Check sheet for the drawn part. Datum: minimum x, y, z corner. Units: mm. A direction names the side the tool comes from. Give positions to 0.01 mm unless a question says otherwise; leave off trailing zeros. Write each loop counter-clockwise with the first axis right and the second up, starting at its lowest first coordinate (ties: lowest second). Pieces come first, ordered by that corner, then holes. Notation, with made-up numbers: (-12, 84.25) - (30, 84.25) arc R36 cw to (30, 118.25) - close; hole circle Ø2 at (-5, 76.25). An arc over 180 degrees is marked (long way). One line per question, with ' | ' between items. Start each with the question number.
Q1. Gauge pin test, flat ends, axial feed: P1, Ø10, axis at x = 37.5, z = 29.5, coming from the +Y side; P2, Ø5, axis at x = 62, z = 22.5, coming from the +Y side; P3, Ø12, axis at x = 248.5, y = 74, coming from the -Z side. Record the tip position at first contact, or that the pin passes through.
Q2. Section check B-B on y = 114.3. Record the boundary of the cut face in (x, z).
Q3. Section check A-A on x = 177.8. Record the boundary of the cut face in (y, z), and give its area (3 significant figures).
Q4. Section check C-C on z = 7. Record the boundary of the cut face in (x, y).
Q5. Section check D-D on x = 129.5. Record the boundary of the cut face in (y, z).
Q6. Thickness scan on L1, parallel to Y at x = 127, z = 42; L2, parallel to X at y = 203, z = 42; L3, parallel to Y at x = 177, z = 41. Record the ranges inside material, lowest first. Write a range as [from, to].
Q7. Set-up check for the marked faces 1 and 2: record each of +Z, -Z, +X, -X, +Y, -Y from which the full face is reachable in a straight line by a thin tool's end or side.
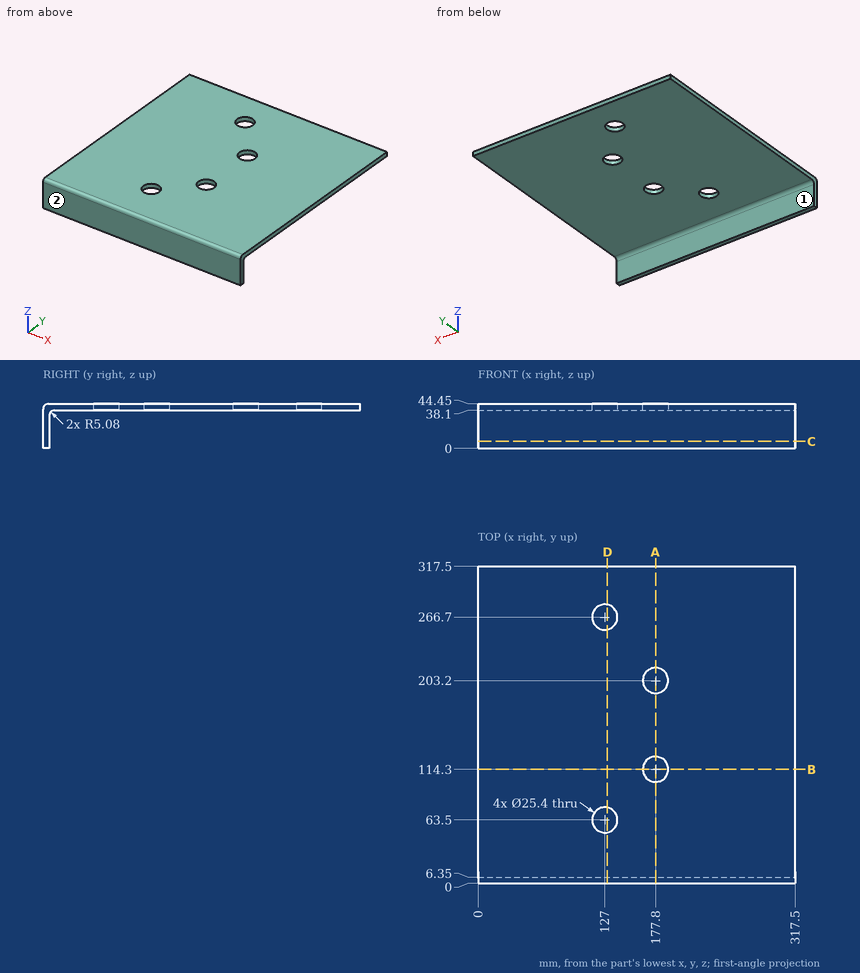
Working result:
1) P1: stops at y = 6.57 | P2: stops at y = 6.35 | P3: stops at z = 38.1
2) outline: (0, 38.1) - (165.1, 38.1) - (165.1, 44.45) - (0, 44.45) - close; (190.5, 38.1) - (317.5, 38.1) - (317.5, 44.45) - (190.5, 44.45) - close
3) outline: (0, 0) - (6.35, 0) - (6.35, 33.02) arc R5.08 cw to (11.43, 38.1) - (101.6, 38.1) - (101.6, 44.45) - (5.08, 44.45) arc R5.08 ccw to (0, 39.37) - close; (127, 38.1) - (190.5, 38.1) - (190.5, 44.45) - (127, 44.45) - close; (215.9, 38.1) - (317.5, 38.1) - (317.5, 44.45) - (215.9, 44.45) - close | area: 1,940 mm2
4) outline: (0, 0) - (317.5, 0) - (317.5, 6.35) - (0, 6.35) - close
5) outline: (0, 0) - (6.35, 0) - (6.35, 33.02) arc R5.08 cw to (11.43, 38.1) - (51.05, 38.1) - (51.05, 44.45) - (5.08, 44.45) arc R5.08 ccw to (0, 39.37) - close; (75.95, 38.1) - (254.25, 38.1) - (254.25, 44.45) - (75.95, 44.45) - close; (279.15, 38.1) - (317.5, 38.1) - (317.5, 44.45) - (279.15, 44.45) - close
6) L1: y = [0.73, 50.8], [76.2, 254], [279.4, 317.5] | L2: x = [0, 165.1], [190.5, 317.5] | L3: y = [0.27, 101.63], [126.97, 190.53], [215.87, 317.5]
7) face 1: -Z, +X, -X, +Y | face 2: +Z, -Z, +X, -X, -Y
